Job drawing, mm, ordinate dimensions from the low corner. One solid piece. Give positions to 0.01 mm unless a question says otherwise; leave off trailing zeros. Loops run counter-clockwise (first coordinate to the right, second up) from the corner with the lowest first, then second, coordinate; pieces in that order, holes last. Notation, with made-up numbers: (54.5, 49.5) - (105.5, 49.5) arc R16 ccw to (105.5, 59.5) - close; hole circle Ø2 at (55, 81). An arc over 180 degrees is marked (long way). Answer as CSV lines item,"result". Start each with the question number.
Item 1: Pin check, flat tips, straight feed: pin 1 (3 mm diameter, centred on x = 12, z = 33, fed in from -Y); pin 2 (10 mm diameter, centred on x = 16, z = 25.5, fed in from +Y); pin 3 (4 mm diameter, centred on y = 8, z = 13, fed in from +X). Stop position of each tip, or through.
Item 2: Saw through at C-C on x = 15.75. Give the cut face in (y, z) (1 decimal).
Item 3: Drill centre lines: L1, parallel to Z at x = 16, y = 8 (1 decimal); L2, parallel to X at y = 7, z = 8 (1 decimal); L3, parallel to Y at x = 15, z = 11.5. Where is each one in solid material? Low to high. Write a range as from..to.
Item 4: Pull direction X, two halves, no side cores. Call the marked faces 1, 2 and 3: pulls with the +X half, pulls with the -X half, needs draft (parallel to the pull), parting line crosses it, or undercut.
Item 5: Saw through at D-D on x = 3.5. Give the cut face in (y, z) (1 decimal).
Item 6: Saw through at A-A on z = 27. Give the cut face in (x, y).
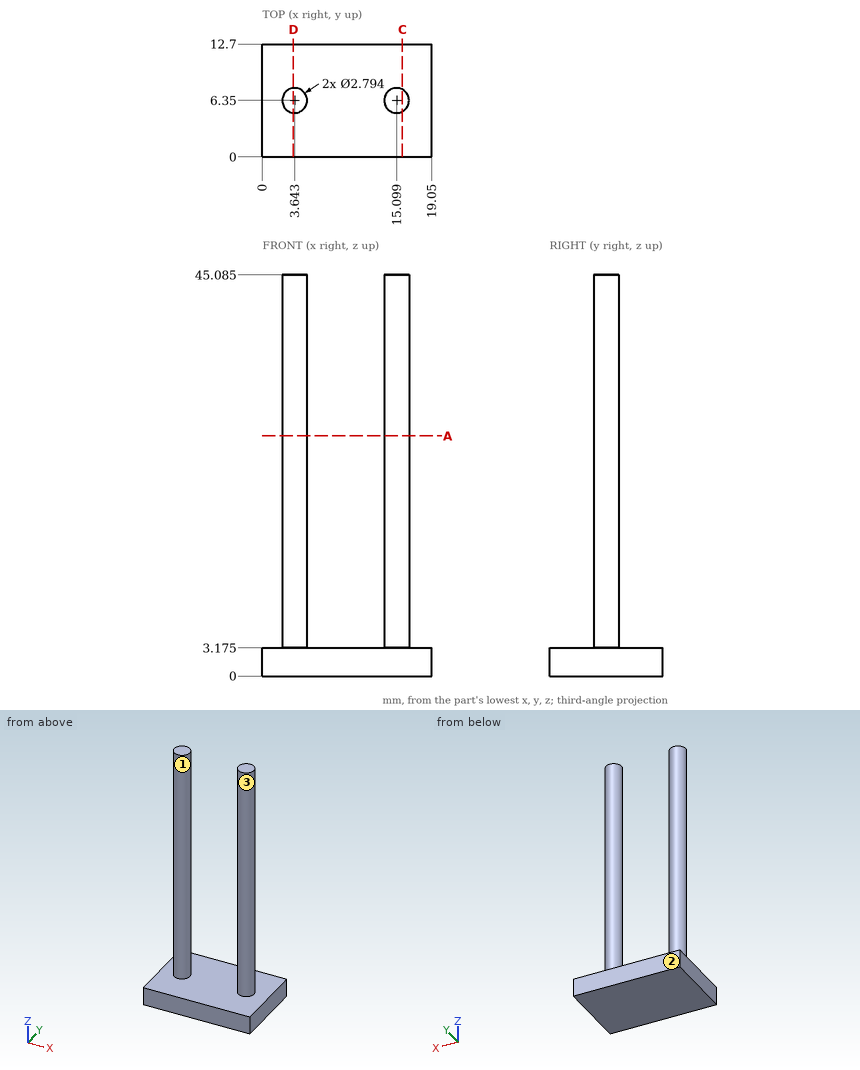
Responses:
1,pin 1,"through"
1,pin 2,"y = 7.75"
1,pin 3,"x = 16.5"
2,outline,"(0, 0) - (12.7, 0) - (12.7, 3.2) - (7.6, 3.2) - (7.6, 45.1) - (5.1, 45.1) - (5.1, 3.2) - (0, 3.2) - close"
3,L1,"0..3.2"
3,L2,"2.4..4.9, 13.9..16.3"
3,L3,"4.96..7.74"
4,face 1,"undercut"
4,face 2,"needs draft"
4,face 3,"undercut"
5,outline,"(0, 0) - (12.7, 0) - (12.7, 3.2) - (7.7, 3.2) - (7.7, 45.1) - (5, 45.1) - (5, 3.2) - (0, 3.2) - close"
6,outline,"circle Ø2.79 at (3.64, 6.35); circle Ø2.79 at (15.1, 6.35)"
